from build123d import *

# Parameters (mm, degrees)
F3_SIZE = 0.5


# Not quite as in the source:
# - a fillet or chamfer that OpenCascade refuses, or shapes differently, is made with other operations: its cross-section is extruded or revolved along the edge and cut away or added


with BuildPart() as f1:
    # F0 (on Front) → F1 (revolve)
    with BuildSketch(Plane.XZ):
        with BuildLine():
            Line((4, 6.25), (0, 6.25))
            Line((0, 6.25), (0, 0.75))
            add(Edge.make_bspline(
                [(10, 0), (10, 0.75), (0, 0.75)],
                knots=[0, 0, 0, 1.5707963268, 1.5707963268, 1.5707963268], degree=2, weights=[1, 0.7071067812, 1]))
            Line((10, 0), (11, 0))
            Line((11, 0), (11, 3))
            Line((11, 3), (6, 3))
            Line((6, 3), (6, 3.75))
            Line((6, 3.75), (4, 3.75))
            Line((4, 3.75), (4, 6.25))
        make_face()
    revolve(axis=Axis((0, 0, 3.5), (0, 0, -1)))

    # F2: fillet of radius 5 on 1 edges, made by hand

    # F2_s1 → F2_t2 (revolve, cut)
    with BuildSketch(Plane.XZ):
        with BuildLine():
            ThreePointArc((10, 0), (10.7434164903, 1.4188611699), (11, 3))
            Line((11, 3), (11, 0))
            Line((11, 0), (10, 0))
        make_face()
    revolve(axis=Axis((0, 0, 0), (0, 0, -1)), mode=Mode.SUBTRACT)

    # F3
    f3_edges = [f1.edges().sort_by_distance(p)[0] for p in [
        (-4, 0, 6.25),
    ]]
    chamfer(f3_edges, length=F3_SIZE)


solid = f1.part
Part model, mm, in its own coordinate system. A direction names the side the tool comes from. Give positions to 0.01 mm unless a question says otherwise; leave off trailing zeros. Use one line per item in the form item = value.
(1) Drill centre lines: line 1 (Y direction, x = 0, z = 5.5); line 2 (Y direction, x = 3.25, z = 2.25); line 3 (X direction, y = -5.25, z = 1.5). Where is each one in solid material? Low to high. Write a range as from..to.
Solution:
line_1 = -4..4
line_2 = -10.45..10.45
line_3 = -9.4..9.4
(2) Flat gauge pins, fed straight in: P1, Ø2, axis at y = 3.5, z = 3, coming from the +X side; P2, Ø1.5, axis at y = 0.5, z = 2, coming from the -X side; P3, Ø2, axis at x = 0.5, y = -5.5, coming from the -Z side. Where does each tip first touch, or does it go through?
Solution:
P1 = 10.71
P2 = -10.99
P3 = 0.57
(3) Tool access for faces 1 (the face through (-0.867, 3.905, 4.764)), 2 (the face through (0, 0, 6.25)): list every direction of +Z, -Z, +X, -X, +Y, -Y with a clear straight run to the whole face (end or side of a thin tool).
Solution:
face_1 = +Z
face_2 = +Z, +X, -X, +Y, -Y
